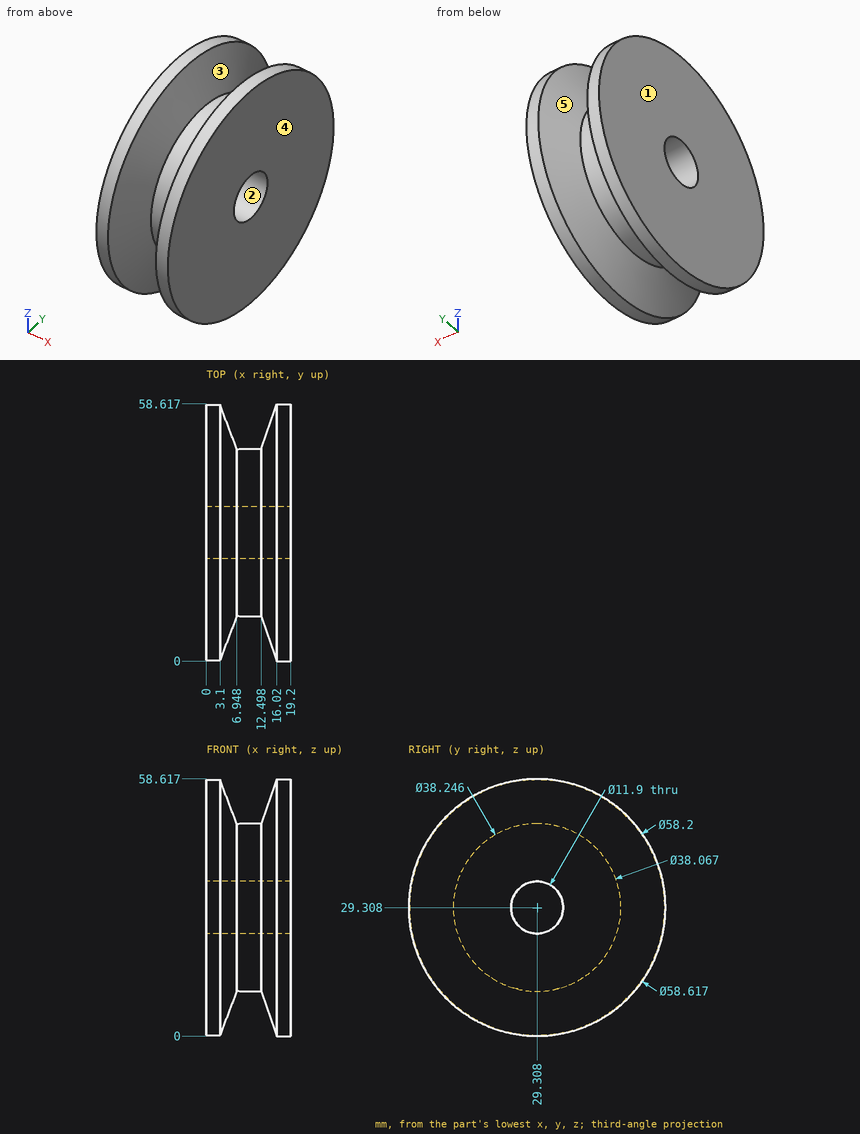
Drawing for the job (mm, zero at the part's lowest x, y, z). A direction names the side the tool comes from. Coordinates: 2 decimals unless noted, no trailing zeros.
Item 1: Two-plate mould, pull along Z, no slides. Class the marked faces 1, 2 and 3: +Z half, -Z half, draft (parallel to the pull), parting line (faces both ways), or undercut.
Check sheet entries:
face 1: draft
face 2: undercut
face 3: parting line
Item 2: Drill centre lines: L1, parallel to Y at x = 1.5, z = 29; L2, parallel to X at y = 8, z = 39 (1 decimal); L3, parallel to X at y = 6, z = 18 (1 decimal). Where is each one in solid material? Low to high.
Check sheet entries:
L1: y = 0.21 to 23.37, 35.25 to 58.41
L2: x = 0 to 5.3, 14 to 19.2
L3: x = 0 to 4.3, 14.8 to 19.2
Item 3: 3-axis set-ups, long thin cutter, end or side, ignore diameter. For the marked faces 4 and 5: which of +Z, -Z, +X, -X, +Y, -Y reach the whole face in a straight line?
Check sheet entries:
face 4: +Z, -Z, +X, +Y, -Y
face 5: none
Item 4: Pin check, flat tips, straight feed: pin 1 Ø2 at (x, y) = (8, 20) entering from -Z (1 decimal); pin 2 Ø6 at (x, z) = (15.5, 25.5) entering from -Y; pin 3 Ø1 at (x, z) = (10.5, 23.5) entering from +Y. Stop position of each tip, or through.
Check sheet entries:
pin 1: stops at z = 12.2
pin 2: stops at y = 0.01
pin 3: stops at y = 47.65
